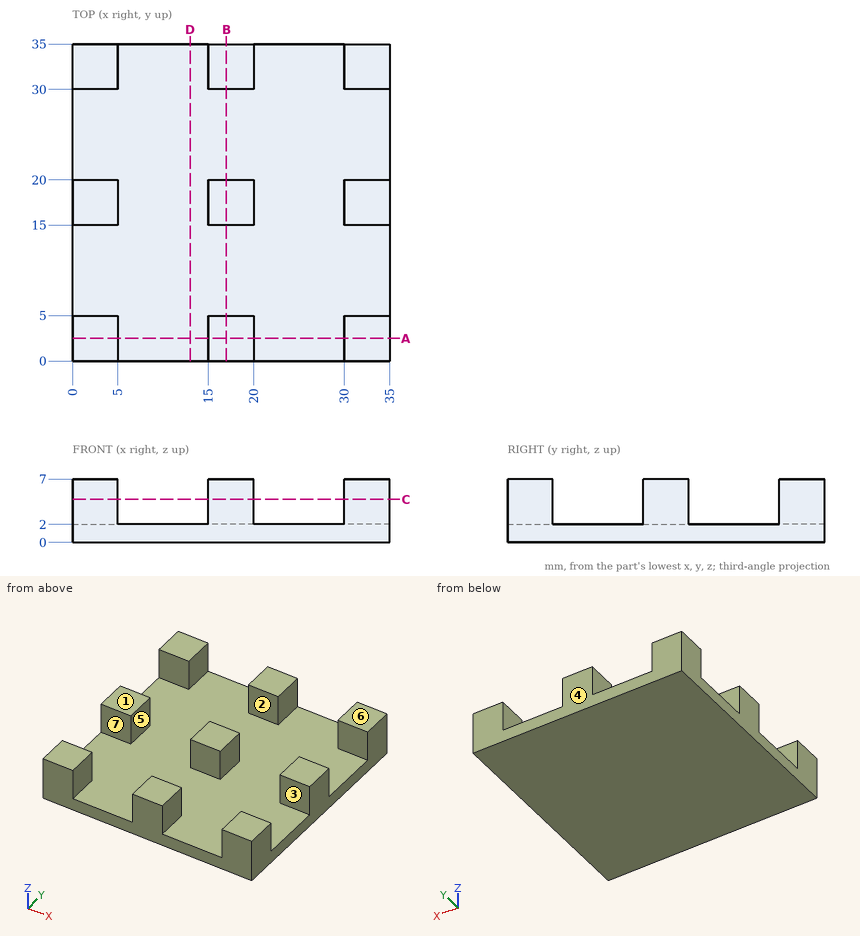
Geometry check sheet. Reference: drawing and pictorial views, mm from the part's lowest x, y, z. A direction names the side the tool comes from. Round coordinates to 2 decimals unless told otherwise and drop trailing zeros. Loops run counter-clockwise (first coordinate to the right, second up) from the corner with the lowest first, then second, coordinate; pieces in that order, holes last. Notation, with made-up numbers: (-24.5, 11.5) -> (3.5, 11.5) arc R12 ccw to (3.5, 32.5) -> close; hole circle Ø7 at (-18.5, -7.75). An arc over 180 degrees is marked (long way). Answer as a JSON object with one key per item and string values. Group by question number.
Item 1: Set-up check for the marked faces 5, 6 and 7: record each of +Z, -Z, +X, -X, +Y, -Y from which the full face is reachable in a straight line by a thin tool's end or side.
Item 2: Release check for a two-part mould opening along Y. For the marked faces 1, 2, 3 and 4 record: pulls with the +Y half, pulls with the -Y half, needs draft (parallel to the pull), parting line crosses it, or undercut.
Item 3: Cross-section at A-A, the plane y = 2.5. Record the cut outline in (x, z), plus the area to 3 significant figures.
Item 4: Cross-section at C-C, the plane z = 4.75. Count the separate pieces of the cut face and the enclosed holes in it, plus the area to 3 significant figures.
Item 5: Cross-section at D-D, the plane x = 13. Record the cut outline in (y, z), plus the area to 3 significant figures.
Item 6: Thickness scan on line 1 along Y through (x, z) = (3.5, 5.75); line 2 along Z through (x, y) = (18, 6.5). Record the ranges inside material, lowest first.
Item 7: Depth check by flat-ended pin: pin 1 Ø1 at (x, y) = (20, 13) entering from +Z; pin 2 Ø2.5 at (y, z) = (3, 4.5) entering from -X; pin 3 Ø1.5 at (y, z) = (6, 3) entering from -X. Enter the tip coordinate at first touch or a pass-through.
Determined:
{
 "1": {"face 5": "+Z, +Y, -Y", "face 6": "+Z, +X, -X, +Y, -Y", "face 7": "+Z, +X, -X"},
 "2": {"face 1": "needs draft", "face 2": "undercut", "face 3": "undercut", "face 4": "pulls with the +Y half"},
 "3": {"outline": "(0, 0) -> (35, 0) -> (35, 7) -> (30, 7) -> (30, 2) -> (20, 2) -> (20, 7) -> (15, 7) -> (15, 2) -> (5, 2) -> (5, 7) -> (0, 7) -> close", "area": "145 mm²"},
 "4": {"separate pieces": "9", "enclosed holes": "0", "area": "225 mm²"},
 "5": {"outline": "(0, 0) -> (35, 0) -> (35, 2) -> (0, 2) -> close", "area": "70.0 mm²"},
 "6": {"line 1": "y = 0 to 5, 15 to 20, 30 to 35", "line 2": "z = 0 to 2"},
 "7": {"pin 1": "stops at z = 2", "pin 2": "stops at x = 0", "pin 3": "passes through"}
}
